Here's how the part is built. I have some questions about the finished solid (model axes, mm). A direction names the side the tool comes from. Give positions to 0.01 mm unless a question says otherwise; leave off trailing zeros. Loops run counter-clockwise (first coordinate to the right, second up) from the corner with the lowest first, then second, coordinate; pieces in that order, holes last. Notation, with made-up numbers: M 87.25,39.5 L 112.25,39.5 A14 ccw 112.25,47.5 Z; hole C 56,49 d6. An arc over 180 degrees is marked long. Answer as CSV lines item,"result". Start each with the question number.
Item 1: If we mould it in two halves opening along Y, with no side actions, what happens to faces 4 (the flat face through (-3, -12, 10)), 5 (the flat face through (-24, 2.9, 4)), 6 (the cylindrical face through (-25.85, -3.77, 2.46))? For each: released by +Y, released by -Y, zero draft, split by the parting line, or undercut.
Item 2: I want a section at A-A on x = -24.5. List the corners of the cut face in (y, z) for me.
Item 3: If I drill on line 1 along Y through (x, z) = (-29, 6); line 2 along Y through (x, z) = (-19.5, 8); line 3 along Z through (x, y) = (-24, 1), over which ranges is the centre line in solid material (lowest first)? Write a range as from..to.
Item 4: For faces 1 (the flat face through (-24, -5, 5)), 2 (the flat face through (-4, -33, 7)), 3 (the flat face through (-11.164, 15, 5)), which set-ups out of +Z, -Z, +X, -X, +Y, -Y let a thin tool reach every point of the face, with its end or its side?
Item 5: I want a section at B-B on z = 4.25. List the corners of the cut face in (x, y) for me.
Item 6: I want a section at C-C on x = -5.5. List the corners of the cut face in (y, z) for me, plus the area to 3 significant figures.
Item 7: I want a section at D-D on x = 0. List the corners of the cut face in (y, z) for me.
Item 8: Will these pins go through, and if not, where does the flat tip stop? P1, Ø3.5, axis at x = -24.5, y = -20, coming from the +Z side; P2, Ø8.5, axis at x = -1.16, y = 10.9, coming from the -Z side; P3, Ø4, axis at x = -30, z = 8, coming from the -Y side.
from build123d import *

# Parameters (mm, degrees)
ESQUISSE1_R             = 3.3
ESQUISSE1_R_2           = 2.75
BOSS_EXTRU_1_DEPTH      = 10
ESQUISSE2_R             = 6
ENL_V_MAT_EXTRU_1_DEPTH = 5
ESQUISSE3_R             = 7
ENL_V_MAT_EXTRU_3_DEPTH = 7


with BuildPart() as part:
    # Esquisse1 → Boss.-Extru.1 (new body)
    with BuildSketch(Plane.XY):
        Polygon((8.835664484, 27.89983396), (8.835664484, -52.10016604), (-11.164335516, -52.10016604), (-11.164335516, -27.10016604), (-36.164335516, -27.10016604), (-36.164335516, 2.89983396), (-11.164335516, 2.89983396), (-11.164335516, 27.89983396), align=None)
        with Locations((-1.164335516, 10.89983396)):
            Circle(ESQUISSE1_R, mode=Mode.SUBTRACT)
        with Locations((-1.164335516, -35.10016604)):
            Circle(ESQUISSE1_R, mode=Mode.SUBTRACT)
        with Locations((-23.664335516, -2.10016604)):
            Circle(ESQUISSE1_R_2, mode=Mode.SUBTRACT)
        with Locations((-23.664335516, -22.10016604)):
            Circle(ESQUISSE1_R_2, mode=Mode.SUBTRACT)
    extrude(amount=BOSS_EXTRU_1_DEPTH)

    # Esquisse2 → Enlèv. mat.-Extru.1 (cut)
    with BuildSketch(Plane.XY.offset(10)):
        with Locations((-23.664335516, -2.10016604)):
            Circle(ESQUISSE2_R)
        with Locations((-23.664335516, -22.10016604)):
            Circle(ESQUISSE2_R)
    extrude(amount=-ENL_V_MAT_EXTRU_1_DEPTH, mode=Mode.SUBTRACT)

    # Esquisse3 → Enlèv. mat.-Extru.3 (cut)
    with BuildSketch(Plane(origin=(0, 0, 0), x_dir=(-1, 0, 0), z_dir=(0, 0, -1))):
        with Locations((1.164335516, 10.89983396)):
            Circle(ESQUISSE3_R)
        with Locations((1.164335516, -35.10016604)):
            Circle(ESQUISSE3_R)
    extrude(amount=-ENL_V_MAT_EXTRU_3_DEPTH, mode=Mode.SUBTRACT)


solid = part.part
Result:
1,face 4,"zero draft"
1,face 5,"released by +Y"
1,face 6,"undercut"
2,outline,"M -27.1,0 L -24.72,0 L -24.72,5 L -27.1,5 Z; M -19.48,0 L -4.72,0 L -4.72,5 L -8.04,5 L -8.04,10 L -16.16,10 L -16.16,5 L -19.48,5 Z; M 0.52,0 L 2.9,0 L 2.9,5 L 0.52,5 Z"
3,line 1,"-27.1..-24.84, -19.36..-4.84, 0.64..2.9"
3,line 2,"-27.1..-26.42, -17.78..-6.42, 2.22..2.9"
3,line 3,"0..5"
4,face 1,"+Z"
4,face 2,"-Z"
4,face 3,"+Z, -Z, -X, +Y"
5,outline,"M -36.16,-27.1 L -11.16,-27.1 L -11.16,-52.1 L 8.84,-52.1 L 8.84,27.9 L -11.16,27.9 L -11.16,2.9 L -36.16,2.9 Z; hole C -23.66,-22.1 d5.5; hole C -23.66,-2.1 d5.5; hole C -1.16,-35.1 d14; hole C -1.16,10.9 d14"
6,outline,"M -52.1,0 L -40.6,0 L -40.6,7 L -29.6,7 L -29.6,0 L 5.4,0 L 5.4,7 L 16.4,7 L 16.4,0 L 27.9,0 L 27.9,10 L -52.1,10 Z"
6,area,"646 mm^2"
7,outline,"M -52.1,0 L -42,0 L -42,7 L -38.19,7 L -38.19,10 L -52.1,10 Z; M -32.01,7 L -28.2,7 L -28.2,0 L 4,0 L 4,7 L 7.81,7 L 7.81,10 L -32.01,10 Z; M 13.99,7 L 17.8,7 L 17.8,0 L 27.9,0 L 27.9,10 L 13.99,10 Z"
8,P1,"z = 5"
8,P2,"z = 7"
8,P3,"y = -27.1"
